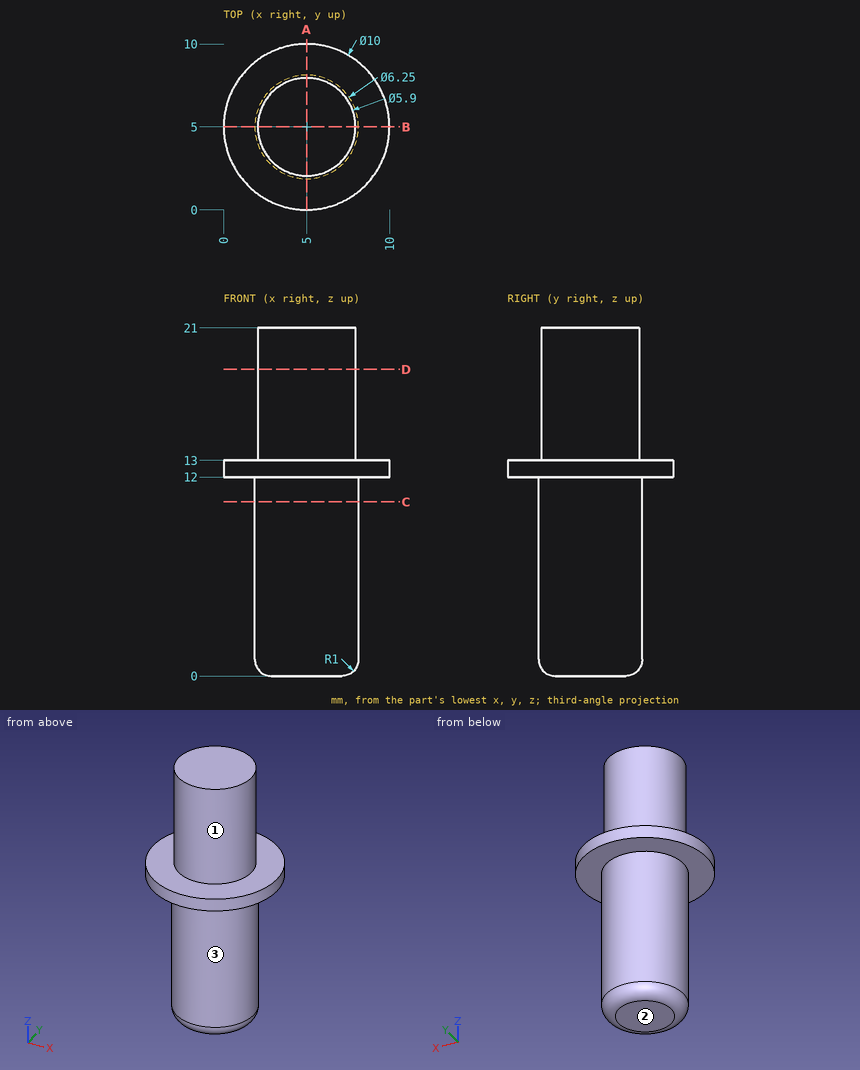
The figure shows three views and two pictorial views of one solid part (mm, origin at its lowest corner). Answer the questions. A direction names the side the tool comes from. Give positions to 0.01 mm unless a question says otherwise; leave off trailing zeros. Write each loop counter-clockwise with the first axis right and the second up, starting at its lowest first coordinate (ties: lowest second). Pieces come first, ordered by that corner, then holes.
Q1. A tool of negligible diameter and unlimited length cuts with its end or side. For the marked faces 1, 2 and 3, from which of +Z, -Z, +X, -X, +Y, -Y can it reach the whole face along a straight path? Write none if from no direction.
Answer:
face 1: +Z
face 2: -Z, +X, -X, +Y, -Y
face 3: -Z
Q2. The part is cut by section C-C on z = 10.5. Give the vertices of the cut face in (x, y) (3 decimals), and give its area (3 significant figures).
Answer:
outline: circle Ø6.25 at (5, 5)
area: 30.7 mm2
Q3. Straight lines are drawn through the part: L1, parallel to Z at x = 4, y = 1; L2, parallel to Z at x = 7.75, y = 6.25; L3, parallel to X at y = 4.5, z = 5. For each, find the intervals that lie inside material, in ascending order.
Answer:
L1: z = 12 to 13
L2: z = 0.56 to 13
L3: x = 1.92 to 8.08
Q4. The part is cut by section A-A on x = 5. Give the vertices of the cut face in (y, z) (3 decimals).
Answer:
outline: (0, 12) - (1.875, 12) - (1.875, 1) arc R1 ccw to (2.875, 0) - (7.125, 0) arc R1 ccw to (8.125, 1) - (8.125, 12) - (10, 12) - (10, 13) - (7.95, 13) - (7.95, 21) - (2.05, 21) - (2.05, 13) - (0, 13) - close
Q5. The part is cut by section D-D on z = 18.5. Give the vertices of the cut face in (x, y).
Answer:
outline: circle Ø5.9 at (5, 5)
Q6. Given pin 1 (3 mm diameter, centred on y = 2.5, z = 13.5, fed in from +X); pin 2 (5 mm diameter, centred on y = 8, z = 13, fed in from -X); pin 3 (3 mm diameter, centred on x = 8.5, y = 8.5, fed in from +Z), each flat-ended and moving along its own axis, determine where each tip first touches the part or whether it passes through.
Answer:
pin 1: stops at x = 9.88
pin 2: stops at x = 0.03
pin 3: stops at z = 13
